from build123d import *

# Parameters (mm, degrees)
F0_W            = 6
F0_H            = 17.5
F3_D            = 6
F4_T            = -2
F6_D            = 8
F6_COPIES_COUNT = 5
F7_SIZE         = 1


# Not quite as in the source:
# - a pattern or mirror of a feature is missing from the dataset's text; its kind, count and spacing are read off the source's solid


with BuildPart() as f1:
    # F0 (on Top) → F1 (revolve)
    with BuildSketch(Plane.XY):
        with Locations((3, 8.75)):
            Rectangle(F0_W, F0_H)
    revolve(axis=Axis((3, 0, 0), (1, 0, 0)))

    # F3 (through all)
    with Locations(Plane(origin=(0, 0, 0), x_dir=(0, 1, 0), z_dir=(-1, 0, 0))):
        with Locations((0, 0)):
            Hole(F3_D / 2)

    # F4
    f4_openings = [f1.faces().sort_by_distance(p)[0] for p in [
        (6, -17.005025, 0),
    ]]
    offset(amount=F4_T, openings=f4_openings)

    # F6 (through all)
    with Locations(Plane(origin=(0, 0, 0), x_dir=(0, 1, 0), z_dir=(-1, 0, 0))):
        with Locations((0, -10)):
            f6 = Hole(F6_D / 2)

    # F6_copies: F6 ×5 about axis
    f6_copies_axis = Axis((0, 0, 0), (1, 0, 0))
    for i in range(1, F6_COPIES_COUNT):
        add(f6.rotate(f6_copies_axis, i * 360 / F6_COPIES_COUNT), mode=Mode.SUBTRACT)

    # F7
    f7_edges = [f1.edges().sort_by_distance(p)[0] for p in [
        (6, -5, 0),
    ]]
    chamfer(f7_edges, length=F7_SIZE)


solid = f1.part
Part model, mm, in its own coordinate system. A direction names the side the tool comes from. Coordinates: 2 decimals unless noted, no trailing zeros. Order: outer loops, then holes, each group sorted by start corner. A loop starts at its lowest first (then second) coordinate and runs counter-clockwise, first axis right, second up. Notation, with made-up numbers: M -15,82 L 13,82 A20 ccw 13,95 Z; hole C -35,-8 d4. An arc over 180 degrees is marked long. One line per question, with ' | ' between items.
Q1. Slice it at A-A (y = 0). Give the cut face in (x, z).
A:
outline: M 0,-17.5 L 6,-17.5 L 6,-15.5 L 2,-15.5 L 2,-5 L 5,-5 L 6,-4 L 6,-3 L 0,-3 Z; M 0,3 L 6,3 L 6,4 L 5,5 L 2,5 L 2,6 L 0,6 Z; M 0,14 L 2,14 L 2,15.5 L 6,15.5 L 6,17.5 L 0,17.5 Z
Q2. Slice it at D-D (z = 0). Give the cut face in (x, y).
A:
outline: M 0,-17.5 L 6,-17.5 L 6,-15.5 L 2,-15.5 L 2,-12.05 L 0,-12.05 Z; M 0,-6.97 L 2,-6.97 L 2,-5 L 5,-5 L 6,-4 L 6,-3 L 0,-3 Z; M 0,3 L 6,3 L 6,4 L 5,5 L 2,5 L 2,6.97 L 0,6.97 Z; M 0,12.05 L 2,12.05 L 2,15.5 L 6,15.5 L 6,17.5 L 0,17.5 Z
Q3. Drill centre lines: line 1 (Y direction, x = 4.3, z = 1); line 2 (Y direction, x = 2.95, z = 2); line 3 (X direction, y = 9.5, z = -4). Where is each one in solid material? Low to high.
A:
line 1: y = -17.47 to -15.47, -4.9 to -2.83, 2.83 to 4.9, 15.47 to 17.47 | line 2: y = -17.39 to -15.37, -4.58 to -2.24, 2.24 to 4.58, 15.37 to 17.39 | line 3: x = 0 to 2
Q4. Slice it at B-B (x = 4.5). Give the cut face in (y, z).
A:
outline: C 0,0 d35; C 0,0 d10; hole C 0,0 d31; hole C 0,0 d6
Q5. Two-plate mould, pull along Y, no slides. Class faces 1 (the face through (3.042, -13.887, -10.648)), 2 (the face through (1.014, 13.492, 3.472)), 3 (the face through (6, 7, -14)): +Y half, -Y half, draft (parallel to the pull), parting line (faces both ways), or undercut.
A:
face 1: parting line | face 2: undercut | face 3: draft
Q6. 3-axis set-ups, long thin cutter, end or side, ignore diameter. For faces 4 (the face through (1.014, -12.956, 5.122)), 5 (the face through (3.52, 1.08, 4.88)): which of +Z, -Z, +X, -X, +Y, -Y reach the whole face in a straight line?
A:
face 4: +X, -X | face 5: +X
Q7. Pin check, flat tips, straight feed: P1, Ø1, axis at x = 4, z = -11, coming from the -Y side; P2, Ø3, axis at y = -11, z = -0.5, coming from the +X side; P3, Ø1.5, axis at x = 3, z = -8.5, coming from the +Y side. Stop position of each tip, or through.
A:
P1: stops at y = -14 | P2: stops at x = 2 | P3: stops at y = 15.69
Q8. Slice it at C-C (z = 10). Give the cut face in (x, y).
A:
outline: M 0,-14.36 L 6,-14.36 L 6,-11.84 L 2,-11.84 L 2,-4 L 0,-4 Z; M 0,4 L 2,4 L 2,11.84 L 6,11.84 L 6,14.36 L 0,14.36 Z
